Check sheet for the drawn part. Datum: minimum x, y, z corner. Units: mm. A direction names the side the tool comes from. Round coordinates to 2 decimals unless told otherwise and drop trailing zeros. Order: outer loops, then holes, each group sorted by start corner. A loop starts at its lowest first (then second) coordinate and runs counter-clockwise, first axis right, second up. Notation, with made-up numbers: (14.25, 37.25) -> (46.25, 37.25) arc R20 ccw to (46.25, 44.25) -> close; hole circle Ø11 at (-17.5, 4.25). An arc over 180 degrees is marked (long way). Answer as a JSON object with one key per item and string values. Group by question number.
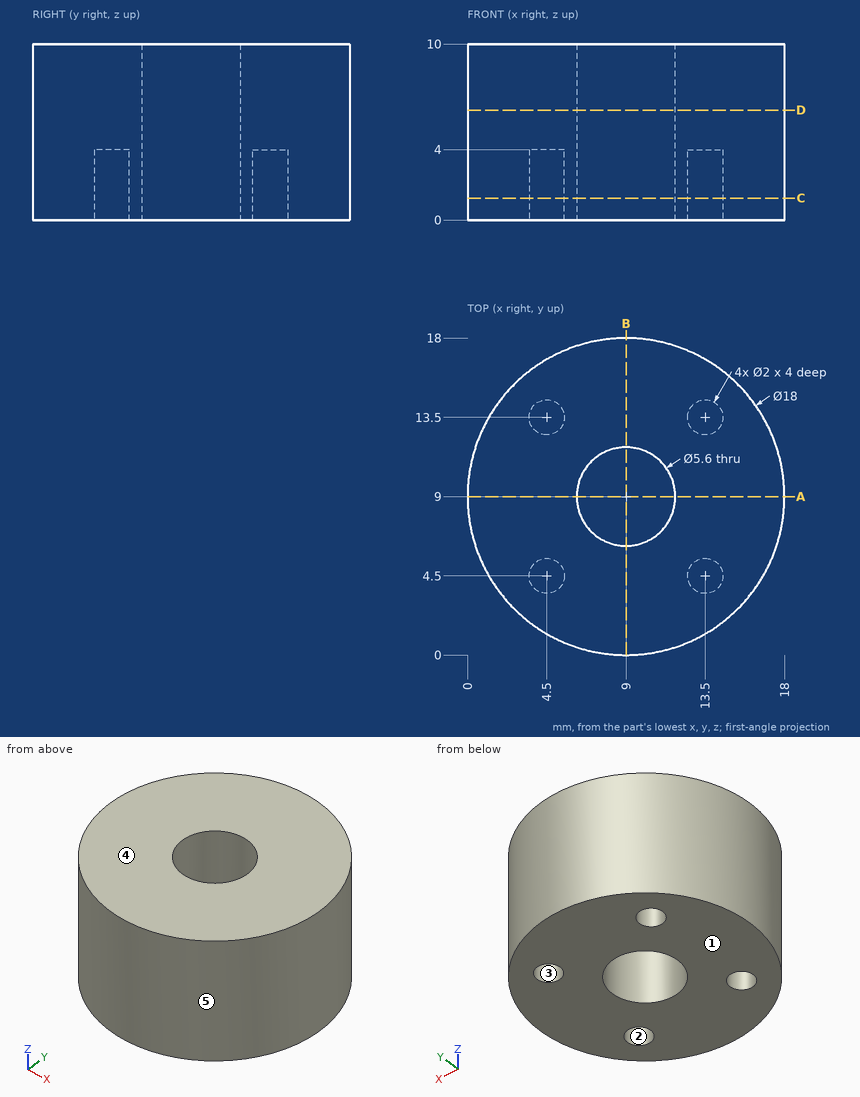
Item 1: Thickness scan on L1, parallel to Y at x = 14.25, z = 2.75; L2, parallel to X at y = 13.5, z = 2.3; L3, parallel to Y at x = 9, z = 6. Record the ranges inside material, lowest first.
Item 2: Sectioned sample at C-C, the plane z = 1.25. Enter the section's corners in (x, y).
Item 3: Sectioned sample at A-A, the plane y = 9. Enter the section's corners in (x, z), then the cut area to 3 significant figures.
Item 4: Sectioned sample at D-D, the plane z = 6.25. Enter the section's corners in (x, y), then the cut area to 3 significant figures.
Item 5: Set-up check for the marked faces 1 and 2: record each of +Z, -Z, +X, -X, +Y, -Y from which the full face is reachable in a straight line by a thin tool's end or side.
Item 6: Depth check by flat-ended pin: pin 1 Ø1 at (x, z) = (12.5, 6) entering from +Y; pin 2 Ø0.6 at (x, y) = (13.5, 4) entering from -Z; pin 3 Ø5 at (x, z) = (3, 8) entering from +Y. Enter the tip coordinate at first touch or a pass-through.
Item 7: Mould release check, pull along X, two halves, no side actions. Record for the marked faces 3, 4 and 5: pulls with the +X half, pulls with the -X half, needs draft (parallel to the pull), parting line crosses it, or undercut.
Result:
{
 "1": {"L1": "y = 1.69 to 3.84, 5.16 to 12.84, 14.16 to 16.31", "L2": "x = 1.21 to 3.5, 5.5 to 12.5, 14.5 to 16.79", "L3": "y = 0 to 6.2, 11.8 to 18"},
 "2": {"outline": "circle Ø18 at (9, 9); hole circle Ø2 at (4.5, 4.5); hole circle Ø2 at (4.5, 13.5); hole circle Ø5.6 at (9, 9); hole circle Ø2 at (13.5, 4.5); hole circle Ø2 at (13.5, 13.5)"},
 "3": {"outline": "(0, 0) -> (6.2, 0) -> (6.2, 10) -> (0, 10) -> close; (11.8, 0) -> (18, 0) -> (18, 10) -> (11.8, 10) -> close", "area": "124 mm2"},
 "4": {"outline": "circle Ø18 at (9, 9); hole circle Ø5.6 at (9, 9)", "area": "230 mm2"},
 "5": {"face 1": "-Z, +X, -X, +Y, -Y", "face 2": "-Z"},
 "6": {"pin 1": "stops at y = 17.49", "pin 2": "stops at z = 4", "pin 3": "stops at y = 17.29"},
 "7": {"face 3": "undercut", "face 4": "needs draft", "face 5": "parting line crosses it"}
}
